Autodesk Inventor part; units mm, degrees
ref_plane "YZ Plane" through (0, 0, 0) normal (1, 0, 0) x (0, 1, 0)
ref_plane "XZ Plane" through (0, 0, 0) normal (0, 1, 0) x (-1, 0, 0)
ref_plane "XY Plane" through (0, 0, 0) normal (0, 0, 1) x (1, 0, 0)
sketch "Sketch1" plane through (0, 0, 0) normal (0, 1, 0) x (-1, 0, 0)
  line L0 (-17.4625, -7.85) -> (-17.4625, -5.31)
  line L1 (-17.4625, -6.35) -> (-17.4625, -5.31)
  line L2 (-17.4625, -5.31) -> (-1.5875, -5.31)
  line L3 (-1.5875, -7.85) -> (-17.4625, -7.85)
  line L4 (-1.5875, -5.31) -> (-1.5875, -0.23)
  line L5 (-1.5875, -7.85) -> (-1.5875, -12.93)
  line L6 (-1.5875, -0.23) -> (30, -0.23)
  line L7 (-1.5875, -12.93) -> (30, -12.93)
  line L8 (30, -12.93) -> (30, -0.23)
  line L9 (61.5875, -7.85) -> (77.4625, -7.85)
  line L10 (77.4625, -5.31) -> (61.5875, -5.31)
  line L11 (77.4625, -7.85) -> (77.4625, -5.31)
  line L12 (77.4625, -6.35) -> (77.4625, -5.31)
  line L13 (61.5875, -7.85) -> (61.5875, -12.93)
  line L14 (61.5875, -5.31) -> (61.5875, -0.23)
  line L15 (61.5875, -0.23) -> (30, -0.23)
  line L16 (61.5875, -12.93) -> (30, -12.93)
  point P0 (-17.4625, -6.58)
  point P1 (77.4625, -6.58)
  dimension "d135" = 6.35
  dimension "d136" = 2.54
extrude "Extrusion1" add sketch "Sketch1" along normal blind 12.7
fillet "Fillet2" radius 6.35 4 edges at (1.5875, 6.35, -12.93) (1.5875, 6.35, -0.23) (-61.5875, 6.35, -12.93) (-61.5875, 6.35, -0.23)
move faces "Move4" translate (25.4, 0, 0) faces at (17.4625, 4.2333, -6.1567)
move faces "Move5" translate (-25.4, 0, 0) faces at (-77.4625, 4.2333, -7.0033)
sketch "Sketch6" plane through (-55.3658, 0, -0.23) normal (0, 0, 1) x (1, 0, 0)
  line L0 (50.7316, 0) -> (0, 0)
  line L1 (56.9533, 0) -> (50.7316, 0)
  ellipse E0 centre (25.3658, 0) end of major axis (56.9533, 0) minor radius 4.7022
  point P0 (55.3658, 0)
extrude "Extrusion18" cut sketch "Sketch6" against normal blind 20.6375
fillet "Fillet4" radius 3.175 2 edges at (-61.5875, 0, -6.58) (1.5875, 0, -6.58)
sketch "Sketch7" plane through (-102.8625, 12.7, -5.31) normal (0, 0, 1) x (1, 0, 0)
  line L0 (41.275, -12.2395) -> (41.275, 0)
  line L1 (41.275, -6.1198) -> (50.8, -6.1198) construction
  line L2 (0, -12.7) -> (0, 0)
  line L3 (41.275, -6.35) -> (47.625, -6.35) construction
  line L4 (98.2283, 0) -> (47.4967, 0)
  line L5 (72.8625, 0) -> (72.8625, -18.9978)
  line L6 (0, -12.7) -> (39.6282, -12.7)
  arc A0 (34.925, -10.4775) -> (34.925, -7.3025) centre (34.925, -8.89) ccw
  line L7 (0, -8.89) -> (6.35, -8.89)
  arc A1 (6.35, -7.3025) -> (6.35, -10.4775) centre (6.35, -8.89) ccw
  line L8 (34.925, -7.3025) -> (6.35, -7.3025)
  line L9 (6.35, -10.4775) -> (34.925, -10.4775)
  arc A2 (110.8, -7.3025) -> (110.8, -10.4775) centre (110.8, -8.89) ccw
  line L10 (145.725, -8.89) -> (139.375, -8.89)
  arc A3 (139.375, -10.4775) -> (139.375, -7.3025) centre (139.375, -8.89) ccw
  line L11 (110.8, -7.3025) -> (139.375, -7.3025)
  line L12 (139.375, -10.4775) -> (110.8, -10.4775)
  point P0 (102.8625, -12.7)
  dimension "d161" = 3.175
  dimension "d162" = 6.35
  dimension "d163" = 3.175
extrude "Extrusion19" cut sketch "Sketch7" against normal blind 20.6375
move faces "Move6" translate (0, -4.7752, 0) faces at (-21.5447, 12.7, -4.4633)
properties part number "AllFretBars"
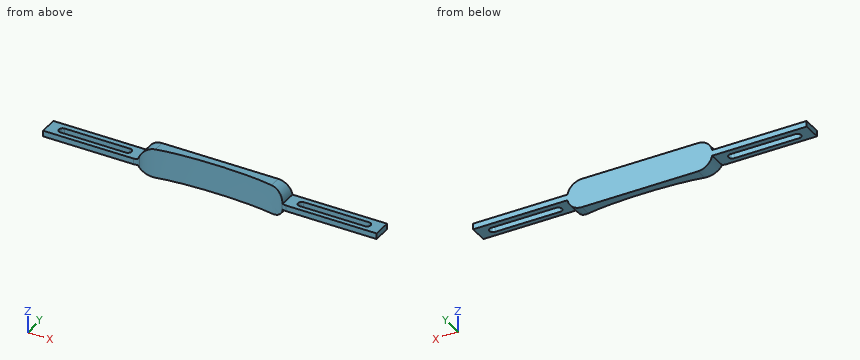
Verification items for the finished model (mm, model axes). Round coordinates to 2 decimals unless told otherwise and drop trailing zeros. Order: outer loops, then holes, each group sorted by start corner. A loop starts at its lowest first (then second) coordinate and runs counter-clockwise, first axis right, second up.
1) Depth check by flat-ended pin: pin 1 (4 mm diameter, centred on x = -82, y = 2, fed in from -Z). Enter the tip coordinate at first touch or a pass-through.
Geometry says:
pin 1: stops at z = -7.85
2) Material ranges on line 1 (Y direction, x = 19, z = -5.5); line 2 (Y direction, x = -29.5, z = -10.25); line 3 (Y direction, x = -12.5, z = -11.75), recorded low to high.
Geometry says:
line 1: y = 0 to 2.22, 5.4 to 7.92
line 2: y = 4.7 to 7.92
line 3: y = 3.91 to 7.92
3) Cross-section at B-B, the plane z = -6.5. Give the number of separate pieces and of enclosed holes in the cut face, plus the area to 3 significant figures.
Geometry says:
separate pieces: 1
enclosed holes: 2
area: 724 mm2
4) Cross-section at A-A, the plane x = 27.5. Record the cut outline in (y, z), plus the area to 3 significant figures.
Geometry says:
outline: (0, -7.85) - (2.22, -7.85) - (2.22, -5.31) - (0, -5.31) - close; (5.4, -7.85) - (7.92, -7.85) - (7.92, -5.31) - (5.4, -5.31) - close
area: 12.1 mm2
